```python
from build123d import *

# Parameters (mm, degrees)
SKETCH1_R           = 15
BOSS_EXTRUDE1_DEPTH = 88
SKETCH2_R           = 2.5
BOSS_EXTRUDE2_DEPTH = 13
BOSS_EXTRUDE3_DEPTH = 18
FILLET1_R           = 4


with BuildPart() as part:
    # Sketch1 → Boss-Extrude1 (new body)
    with BuildSketch(Plane(origin=(0, 0, 0), x_dir=(1, 0, 0), z_dir=(0, 1, 0))):
        Circle(SKETCH1_R)
    extrude(amount=BOSS_EXTRUDE1_DEPTH)

    # Sketch2 → Boss-Extrude2 (add)
    with BuildSketch(Plane(origin=(0, 88, 0), x_dir=(1, 0, 0), z_dir=(0, 1, 0))):
        Circle(SKETCH2_R)
    extrude(amount=BOSS_EXTRUDE2_DEPTH)

    # Sketch3 → Boss-Extrude3 (add)
    with BuildSketch(Plane(origin=(0, 18, 0), x_dir=(-1, 0, 0), z_dir=(0, -1, 0))):
        with BuildLine():
            Line((0, 15), (25, 15))
            Line((25, 15), (25, -15))
            Line((25, -15), (0, -15))
            ThreePointArc((0, -15), (-15, 0), (0, 15))
        make_face()
    extrude(amount=BOSS_EXTRUDE3_DEPTH)

    # Fillet1
    fillet1_edges = [part.edges().sort_by_distance(p)[0] for p in [
        (-25, 9, -15),
        (-25, 9, 15),
    ]]
    fillet(fillet1_edges, radius=FILLET1_R)


solid = part.part
```
Design review of the part built by this model. Coordinates are the model's own, in mm. A direction names the side the tool comes from. Give positions to 0.01 mm unless a question says otherwise; leave off trailing zeros. Loops run counter-clockwise (first coordinate to the right, second up) from the corner with the lowest first, then second, coordinate; pieces in that order, holes last. Notation, with made-up numbers: (-3, 58.5) -> (13, 58.5) arc R26 cw to (13, 88.5) -> close; hole circle Ø2 at (60, 85). An arc over 180 degrees is marked (long way). Write each question's results on one line, items separated by ' | '.
Q1. Take a section at C-C, the plane x = -5.5. Write out the cut boundary in (y, z).
Reply:
outline: (0, -15) -> (18, -15) -> (18, -13.96) -> (88, -13.96) -> (88, 13.96) -> (18, 13.96) -> (18, 15) -> (0, 15) -> close
Q2. Take a section at A-A, the plane z = 0. Write out the cut boundary in (x, y).
Reply:
outline: (-25, 0) -> (15, 0) -> (15, 88) -> (2.5, 88) -> (2.5, 101) -> (-2.5, 101) -> (-2.5, 88) -> (-15, 88) -> (-15, 18) -> (-25, 18) -> close
Q3. For pin 1 Ø6 at (y, z) = (23, -9) entering from +X; pin 2 Ø5 at (x, y) = (-15, 71.5) entering from +Z; pin 3 Ø8 at (x, y) = (9.5, 55.5) entering from -Z; pin 4 Ø12 at (x, z) = (-0.5, -7) entering from -Y, all flat-tipped, find the tip position at first contact; note any pin that passes through.
Reply:
pin 1: stops at x = 13.75 | pin 2: stops at z = 8.29 | pin 3: stops at z = -13.96 | pin 4: stops at y = 0
Q4. Machinability: for faces 1 (the face through (-10, 9, -15)), 2 (the face through (-0.54, 94.41, 2.44)), which of the approach directions +Z, -Z, +X, -X, +Y, -Y give a long, thin tool a straight path to every point of the face, cutting with its end or side? Answer none if there is none.
Reply:
face 1: -Z, +X, -X, +Y, -Y | face 2: +Y
Q5. Wall thickness on L1, parallel to Y at x = -18, z = -7.5; L2, parallel to Y at x = -3, z = -3.25; L3, parallel to Z at x = -8, y = 55: over which ranges is each line inside the solid? List them lowest first.
Reply:
L1: y = 0 to 18 | L2: y = 0 to 88 | L3: z = -12.69 to 12.69
Q6. Take a section at B-B, the plane y = 22. Write out the cut boundary in (x, z).
Reply:
outline: circle Ø30 at (0, 0)
Q7. Take a section at D-D, the plane x = -16. Write out the cut boundary in (y, z), plus the area to 3 significant figures.
Reply:
outline: (0, -15) -> (18, -15) -> (18, 15) -> (0, 15) -> close | area: 540 mm²
